Build history of the part. All positions in model axes, mm. Give positions to 0.01 mm unless a question says otherwise; leave off trailing zeros. Loops run counter-clockwise (first coordinate to the right, second up) from the corner with the lowest first, then second, coordinate; pieces in that order, holes last. Notation, with made-up numbers: (13, 45.25) -> (22, 45.25) arc R19 ccw to (22, 57.25) -> close; hole circle Ø9 at (84.5, 25.5). An arc over 180 degrees is marked (long way). Answer in a Markdown table with one row per item. Add a question column.
from build123d import *

# Parameters (mm, degrees)
F0_W        = 40
F0_H        = 20
F0_R        = 1.75
F0_R_2      = 2.5
F0_R_3      = 2
F0_R_4      = 1.7
F0_R_5      = 2.35
F0_R_6      = 3.5
F0_R_7      = 3.3
F0_R_8      = 1.9586185138
F0_R_9      = 3
F0_R_10     = 2.8292671529
F1_DEPTH    = 4
F2_T1_DEPTH = 25
F2_T3_DEPTH = 45


# Not quite as in the source:
# - a fillet or chamfer that OpenCascade refuses, or shapes differently, is made with other operations: its cross-section is extruded or revolved along the edge and cut away or added


with BuildPart() as f1:
    # F0 (on Front) → F1 (new body)
    with BuildSketch(Plane.XZ):
        with Locations((20, 10)):
            Rectangle(F0_W, F0_H)
        with Locations((19.0599078035, 2.4311765472)):
            Circle(F0_R, mode=Mode.SUBTRACT)
        with Locations((12.9404438354, 4.3140889982)):
            Circle(F0_R_2, mode=Mode.SUBTRACT)
        with Locations((3.878928961, 5.1378629939)):
            Circle(F0_R_3, mode=Mode.SUBTRACT)
        with Locations((23.6495067011, 3.1372687739)):
            Circle(F0_R_4, mode=Mode.SUBTRACT)
        with Locations((29.0628805159, 3.7256787709)):
            Circle(F0_R_2, mode=Mode.SUBTRACT)
        with Locations((36.1237967933, 3.8433607703)):
            Circle(F0_R_5, mode=Mode.SUBTRACT)
        with Locations((20.3544088753, 9.6097794314)):
            Circle(F0_R_6, mode=Mode.SUBTRACT)
        with Locations((9.8807118513, 13.6109674106)):
            Circle(F0_R_7, mode=Mode.SUBTRACT)
        with Locations((2.8197907362, 17.1414283137)):
            Circle(F0_R_8, mode=Mode.SUBTRACT)
        with Locations((17.1769958133, 16.9060624719)):
            Circle(F0_R_2, mode=Mode.SUBTRACT)
        with Locations((31.5342015816, 10.9042814246)):
            Circle(F0_R_9, mode=Mode.SUBTRACT)
        with Locations((25.5324186913, 16.3176533965)):
            Circle(F0_R_10, mode=Mode.SUBTRACT)
        with Locations((35.1823444841, 15.2585163235)):
            Circle(F0_R_3, mode=Mode.SUBTRACT)
    extrude(amount=F1_DEPTH)

    # F2: fillet of radius 1 on 8 edges, made by hand

    # F2_s2 → F2_t1 (cut)
    with BuildSketch(Plane.XY.offset(-2.5)):
        with BuildLine():
            ThreePointArc((0, -3), (0.2928932188, -3.7071067812), (1, -4))
            Line((1, -4), (0, -4))
            Line((0, -4), (0, -3))
        make_face()
        with BuildLine():
            ThreePointArc((40, -3), (39.7071067812, -3.7071067812), (39, -4))
            Line((39, -4), (40, -4))
            Line((40, -4), (40, -3))
        make_face()
        with BuildLine():
            ThreePointArc((0, -1), (0.2928932188, -0.2928932188), (1, 0))
            Line((1, 0), (0, 0))
            Line((0, 0), (0, -1))
        make_face()
        with BuildLine():
            ThreePointArc((40, -1), (39.7071067812, -0.2928932188), (39, 0))
            Line((39, 0), (40, 0))
            Line((40, 0), (40, -1))
        make_face()
    extrude(amount=F2_T1_DEPTH, mode=Mode.SUBTRACT)

    # F2_s4 → F2_t3 (cut)
    with BuildSketch(Plane.YZ.offset(-2.5)):
        with BuildLine():
            ThreePointArc((-3, 20), (-3.7071067812, 19.7071067812), (-4, 19))
            Line((-4, 19), (-4, 20))
            Line((-4, 20), (-3, 20))
        make_face()
        with BuildLine():
            ThreePointArc((-3, 0), (-3.7071067812, 0.2928932188), (-4, 1))
            Line((-4, 1), (-4, 0))
            Line((-4, 0), (-3, 0))
        make_face()
        with BuildLine():
            ThreePointArc((-1, 20), (-0.2928932188, 19.7071067812), (0, 19))
            Line((0, 19), (0, 20))
            Line((0, 20), (-1, 20))
        make_face()
        with BuildLine():
            ThreePointArc((-1, 0), (-0.2928932188, 0.2928932188), (0, 1))
            Line((0, 1), (0, 0))
            Line((0, 0), (-1, 0))
        make_face()
    extrude(amount=F2_T3_DEPTH, mode=Mode.SUBTRACT)


solid = f1.part
(1) Two-plate mould, pull along X, no slides. Class faces 1 (the flat face through (20, -2, 20)), 2 (the cylindrical face through (39.715, -3.699, 9.86)), 3 (the cylindrical face through (28.23, -1.97, 17.17)): released by +X, released by -X, zero draft, split by the parting line, or undercut.
(2) Wall check: line 1 along X through (y, z) = (-0.9, 17); line 2 along X through (y, z) = (-0.35, 5.5); line 3 along X through (y, z) = (-3.75, 11.25). Give the ranges that are in metal, low to high. Write a range as from..to.
(3) Saw through at D-D, the plane x = 21.5. List the corners of the cut face in (y, z), then the cut area to 3 significant figures.
(4) Saw through at B-B, the plane y = -3.5. State how many separate pieces and enclosed holes the cut face has, then the cut area to 3 significant figures.
(5) Saw through at C-C, the plane z = 11.5. List the corners of the cut face in (x, y).
(6) Flat gauge pins, fed straight in: pin 1 Ø5.5 at (x, z) = (31.53, 10.9) entering from -Y; pin 2 Ø6 at (x, z) = (29.06, 3.73) entering from -Y. Where does each tip first touch, or does it go through?
(7) Saw through at A-A, the plane x = 29. List the corners of the cut face in (y, z).
Worked answers:
| question | item | result |
|---|---|---|
| 1 | face 1 | zero draft |
| 1 | face 2 | released by +X |
| 1 | face 3 | undercut |
| 2 | line 1 | 0.01..0.87, 4.77..14.68, 19.68..22.79, 28.28..34.2, 36.17..39.99 |
| 2 | line 2 | 0.24..1.91, 5.85..10.74, 15.14..27.3, 30.82..34.46, 37.79..39.76 |
| 2 | line 3 | 0.34..7.58, 12.19..17.26, 23.45..28.55, 34.51..39.66 |
| 3 | outline | (-4, 1) arc R1 ccw to (-3, 0) -> (-1, 0) arc R1 ccw to (0, 1) -> (0, 6.3) -> (-4, 6.3) -> close; (-4, 12.92) -> (0, 12.92) -> (0, 19) arc R1 ccw to (-1, 20) -> (-3, 20) arc R1 ccw to (-4, 19) -> close |
| 3 | area | 52.7 mm^2 |
| 4 | separate pieces | 1 |
| 4 | enclosed holes | 13 |
| 4 | area | 526 mm^2 |
| 5 | outline | (0, -3) arc R1 ccw to (1, -4) -> (7.34, -4) -> (7.34, 0) -> (1, 0) arc R1 ccw to (0, -1) -> close; (12.42, -4) -> (17.41, -4) -> (17.41, 0) -> (12.42, 0) -> close; (23.3, -4) -> (28.59, -4) -> (28.59, 0) -> (23.3, 0) -> close; (34.47, -4) -> (39, -4) arc R1 ccw to (40, -3) -> (40, -1) arc R1 ccw to (39, 0) -> (34.47, 0) -> close |
| 6 | pin 1 | through |
| 6 | pin 2 | y = -4 |
| 7 | outline | (-4, 1) arc R1 ccw to (-3, 0) -> (-1, 0) arc R1 ccw to (0, 1) -> (0, 1.23) -> (-4, 1.23) -> close; (-4, 6.22) -> (0, 6.22) -> (0, 9.3) -> (-4, 9.3) -> close; (-4, 12.51) -> (0, 12.51) -> (0, 19) arc R1 ccw to (-1, 20) -> (-3, 20) arc R1 ccw to (-4, 19) -> close |
